```python
from build123d import *

# Parameters (mm, degrees)
BOSS_EXTRUDE1_DEPTH = 50
CHAMFER1_SIZE       = 10
SKETCH2_R           = 4
CUT_EXTRUDE1_DEPTH  = 80
SKETCH3_R           = 11
SKETCH3_R_2         = 8
BOSS_EXTRUDE2_DEPTH = 5
SKETCH4_W           = 12
SKETCH4_H           = 12
BOSS_EXTRUDE3_DEPTH = 350
SKETCH5_W           = 46
SKETCH5_H           = 12
BOSS_EXTRUDE4_DEPTH = 12
SKETCH9_W           = 11
SKETCH9_H           = 11
CUT_EXTRUDE3_DEPTH  = 380
BOSS_EXTRUDE5_DEPTH = 10
FILLET1_R           = 3
BOSS_EXTRUDE6_DEPTH = 20
FILLET2_R           = 3
SKETCH12_R          = 10
SKETCH12_R_2        = 2
CUT_EXTRUDE5_DEPTH  = 10


with BuildPart() as part:
    # Sketch1 → Boss-Extrude1 (new body)
    with BuildSketch(Plane.XY):
        Polygon((-65.816488176, 13.044356197), (-65.816488176, -46.955643803), (4.183511824, -46.955643803), (4.183511824, 13.044356197), (2.683511824, 13.044356197), (2.683511824, -45.455643803), (-64.316488176, -45.455643803), (-64.316488176, 13.044356197), align=None)
    extrude(amount=BOSS_EXTRUDE1_DEPTH)

    # Chamfer1
    chamfer1_edges = [part.edges().sort_by_distance(p)[0] for p in [
        (-65.066488176, 13.044356197, 0),
        (3.433511824, 13.044356197, 50),
        (-65.066488176, 13.044356197, 50),
        (3.433511824, 13.044356197, 0),
    ]]
    chamfer(chamfer1_edges, length=CHAMFER1_SIZE)

    # Sketch2 → Cut-Extrude1 (cut)
    with BuildSketch(Plane(origin=(4.183511824, 0, 0), x_dir=(0, 0, -1), z_dir=(1, 0, 0))):
        with Locations((-25, -6.955643803)):
            Circle(SKETCH2_R)
    extrude(amount=-CUT_EXTRUDE1_DEPTH, mode=Mode.SUBTRACT)

    # Sketch3 → Boss-Extrude2 (add)
    with BuildSketch(Plane(origin=(4.183511824, 0, 0), x_dir=(0, 0, -1), z_dir=(1, 0, 0))):
        with Locations(Location((-25, -6.955643803, 0), (0, 0, 180))):
            Circle(SKETCH3_R)
        with Locations((-25, -6.955643803)):
            Circle(SKETCH3_R_2, mode=Mode.SUBTRACT)
    boss_extrude2 = extrude(amount=BOSS_EXTRUDE2_DEPTH)

    # Mirror1: Boss-Extrude2 across plane
    add(boss_extrude2.mirror(Plane.ZY.offset(30.816488176)))

    # Sketch4 → Boss-Extrude3 (add)
    with BuildSketch(Plane(origin=(0, 0, 0), x_dir=(-1, 0, 0), z_dir=(0, 0, -1))):
        with Locations((1.816488176, -52.955643803)):
            Rectangle(SKETCH4_W, SKETCH4_H)
    boss_extrude3 = extrude(amount=-BOSS_EXTRUDE3_DEPTH)

    # Mirror2: Boss-Extrude3 across plane
    add(boss_extrude3.mirror(Plane.ZY.offset(30.816488176)))

    # Sketch5 → Boss-Extrude4 (add)
    with BuildSketch(Plane(origin=(0, 0, 0), x_dir=(-1, 0, 0), z_dir=(0, 0, -1))):
        with Locations((30.816488176, -52.955643803)):
            Rectangle(SKETCH5_W, SKETCH5_H)
    extrude(amount=-BOSS_EXTRUDE4_DEPTH)

    # Sketch9 → Cut-Extrude3 (cut)
    with BuildSketch(Plane.XY.offset(350)):
        with Locations((-59.816488176, -52.955643803)):
            Rectangle(SKETCH9_W, SKETCH9_H)
    cut_extrude3 = extrude(amount=-CUT_EXTRUDE3_DEPTH, mode=Mode.SUBTRACT)

    # Mirror3: Cut-Extrude3 across plane
    add(cut_extrude3.mirror(Plane.ZY.offset(30.816488176)), mode=Mode.SUBTRACT)

    # Sketch10 → Boss-Extrude5 (add)
    with BuildSketch(Plane(origin=(-53.816488176, 0, 0), x_dir=(0, 0, -1), z_dir=(1, 0, 0))):
        Polygon((-35.237542048, -45.455643803), (-65, -45.455643803), (-65, -30.455643803), (-64, -30.455643803), (-64, -44.455643803), (-35.237542048, -44.455643803), align=None)
    extrude(amount=BOSS_EXTRUDE5_DEPTH)

    # Fillet1
    fillet1_edges = [part.edges().sort_by_distance(p)[0] for p in [
        (-53.816488176, -30.455643803, 64.5),
        (-43.816488176, -30.455643803, 64.5),
    ]]
    fillet(fillet1_edges, radius=FILLET1_R)

    # Sketch11 → Boss-Extrude6 (add)
    with BuildSketch(Plane.XY.offset(50)):
        Polygon((-65.816488176, -45.345911858), (-53.816488176, -45.455643803), (-53.816488176, 54.544356197), (-54.816488176, 54.544356197), (-54.816488176, -44.446457666), (-65.840689421, -44.345648745), align=None)
    extrude(amount=BOSS_EXTRUDE6_DEPTH)

    # Fillet2
    fillet2_edges = [part.edges().sort_by_distance(p)[0] for p in [
        (-54.316488176, 54.544356197, 50),
        (-54.316488176, 54.544356197, 70),
    ]]
    fillet(fillet2_edges, radius=FILLET2_R)

    # Sketch12 → Cut-Extrude5 (cut)
    with BuildSketch(Plane(origin=(-53.816488176, 0, 0), x_dir=(0, 0, -1), z_dir=(1, 0, 0))):
        with Locations((-75, 29.544356197)):
            Circle(SKETCH12_R)
        with Locations((-63.5, 41.044356197)):
            Circle(SKETCH12_R_2)
        with Locations((-63.5, 18.044356197)):
            Circle(SKETCH12_R_2)
    extrude(amount=-CUT_EXTRUDE5_DEPTH, mode=Mode.SUBTRACT)


solid = part.part
```
Check sheet for the modelled part. Datum: model origin and axes. Units: mm. A direction names the side the tool comes from. Round coordinates to 2 decimals unless told otherwise and drop trailing zeros. Loops run counter-clockwise (first coordinate to the right, second up) from the corner with the lowest first, then second, coordinate; pieces in that order, holes last. Notation, with made-up numbers: (-16.5, -1) - (21.5, -1) arc R19 cw to (21.5, 6) - close; hole circle Ø4 at (2, -34). An arc over 180 degrees is marked (long way). Answer as a JSON object with one key per item and string values. Group by question number.
Q1. Scan lines: line 1 along X through (y, z) = (-47, 296.5); line 2 along X through (y, z) = (0.5, 15); line 3 along Y through (x, z) = (-69, 25). Record each from-to range of solid material in increasing order. Write a range as [from, to].
Q2. Gauge pin test, flat ends, axial feed: P1, Ø6, axis at x = -60.5, z = 270.5, coming from the +Y side; P2, Ø0.8, axis at x = 3, z = 27.5, coming from the +Y side; P3, Ø4, axis at x = -60.5, y = -39, coming from the -Z side; P4, Ø3.5, axis at y = -55.5, z = 170, coming from the +X side. Record the tip position at first contact, or that the pin passes through.
Q3. Set-up check for faces 1 (the face through (-60, -47.456, 177)), 2 (the face through (2.684, -16, 25)), 3 (the face through (6.65, -10.26, 35.49)): record each of +Z, -Z, +X, -X, +Y, -Y from which the full face is reachable in a straight line by a thin tool's end or side.
Q4. Sectioned sample at A-A, the plane z = 126. Enter the section's corners in (x, y), plus the area to 3 significant figures.
Q5. Mould release check, pull along Z, two halves, no side actions. Record for faces 4 (the face through (-65.056, 7.974, 45.07)), 5 (the face through (3.444, -9.39, 28.174)), 6 (the face through (-30, -45.456, 25)): released by +Z, released by -Z, zero draft, split by the parting line, or undercut.
Q6. Sectioned sample at B-B, the plane z = 25. Count the separate pieces of the cut face and the enclosed holes in it, plus the area to 4 significant figures.
Solution:
{
 "1": {"line 1": "x = [-65.82, -53.82], [-7.82, 4.18]", "line 2": "x = [-65.82, -64.32], [2.68, 4.18]", "line 3": "y = [-17.96, -14.96], [1.04, 4.04]"},
 "2": {"P1": "stops at y = -46.96", "P2": "stops at y = 13.04", "P3": "passes through", "P4": "stops at x = 4.18"},
 "3": {"face 1": "+Z, -Z", "face 2": "+Z, -Z, +Y", "face 3": "+X"},
 "4": {"outline": "(-65.82, -58.96) - (-53.82, -58.96) - (-53.82, -46.96) - (-65.82, -46.96) - close; (-7.82, -58.96) - (4.18, -58.96) - (4.18, -46.96) - (-7.82, -46.96) - close; hole (-65.32, -58.46) - (-54.32, -58.46) - (-54.32, -47.46) - (-65.32, -47.46) - close; hole (-7.32, -58.46) - (3.68, -58.46) - (3.68, -47.46) - (-7.32, -47.46) - close", "area": "46.0 mm²"},
 "5": {"face 4": "released by +Z", "face 5": "undercut", "face 6": "zero draft"},
 "6": {"separate pieces": "3", "enclosed holes": "2", "area": "362.5 mm²"}
}
